Can you work these out from the model? Positions are in its coordinate system, mm. Face numbers are marked on the shaded views. A direction names the side the tool comes from. Round coordinates to 2 decimals unless told otherwise and drop trailing zeros. Write each loop counter-clockwise with the first axis right and the second up, starting at its lowest first coordinate (ties: lowest second). Pieces come first, ordered by that corner, then holes. Notation, with made-up numbers: M -31.5,-4.5 L 21.5,-4.5 A21 ccw 21.5,26.5 Z; hole C 56.25,59 d8. An arc over 180 degrees is marked long. Answer as a JSON object with one key per item and string values. Group by question number.
1) Suppose I cut it at C-C, the plane x = 2.25. Write out the boundary of the cut face in (y, z).
2) On a 3-axis mill with a long thin cutter (end or side, diameter ignored), from which of +Z, -Z, +X, -X, +Y, -Y can I reach the whole of each face in a straight line? I mean the marked faces 1 and 2. Say none if no direction works.
3) Suppose I cut it at D-D, the plane z = -1. Write out the boundary of the cut face in (x, y).
4) Please list where these lines run through material, in increasing order: L1, parallel to X at y = 0.75, z = -9.75; L2, parallel to Z at x = 2, y = 2.05; L3, parallel to Y at x = 8, z = -2.5. Write a range as [from, to].
5) Suppose I cut it at A-A, the plane z = -4.75. Write out the boundary of the cut face in (x, y).
6) Suppose I cut it at B-B, the plane x = 11.25. Write out the boundary of the cut face in (y, z), and give its area (3 significant figures).
7) I'm going to push flat-ended pins straight in: pin 1 Ø1.8 at (x, y) = (1, 2.5) entering from +Z; pin 2 Ø0.8 at (x, z) = (-0.5, -4.5) entering from -Y; pin 3 Ø5 at (x, z) = (10.5, -3.5) entering from +Y. Where does each tip first touch, or does it pass through?
from build123d import *

# Parameters (mm, degrees)
SKETCH1_R           = 0.5
SKETCH1_W           = 6.5
SKETCH1_H           = 9.1
BOSS_EXTRUDE1_DEPTH = 1
BOSS_EXTRUDE2_START = 1
SKETCH1_3_W         = 1
SKETCH1_3_H         = 9.1
SKETCH1_3_W_2       = 6.5
BOSS_EXTRUDE2_DEPTH = 3.2
FILLET1_R           = 1


with BuildPart() as part:
    # Sketch1 → Boss-Extrude1 (new body)
    # profile 1 of 2: a face of its own
    with BuildSketch(Plane(origin=(0, 0, 0), x_dir=(1, 0, 0), z_dir=(0, 1, 0))):
        Polygon((0, 1.45), (0, 0), (13.75, 0), (13.75, 12), (0, 12), (0, 10.55), (6.5, 10.55), (6.5, 1.45), align=None)
        with Locations(Location((11.25, 2.25, 0), (0, 0, 270))):
            Circle(SKETCH1_R, mode=Mode.SUBTRACT)
        with Locations(Location((11.25, 4.75, 0), (0, 0, 270))):
            Circle(SKETCH1_R, mode=Mode.SUBTRACT)
        with Locations(Location((11.25, 7.25, 0), (0, 0, 270))):
            Circle(SKETCH1_R, mode=Mode.SUBTRACT)
        with Locations(Location((11.25, 9.75, 0), (0, 0, 270))):
            Circle(SKETCH1_R, mode=Mode.SUBTRACT)
    # profile 2 of 2: a face of its own
    with BuildSketch(Plane(origin=(0, 0, 0), x_dir=(1, 0, 0), z_dir=(0, 1, 0))):
        with Locations((3.25, 6)):
            Rectangle(SKETCH1_W, SKETCH1_H)
    extrude(amount=BOSS_EXTRUDE1_DEPTH)

    # Sketch1<3> → Boss-Extrude2 (add)
    with BuildSketch(Plane(origin=(0, 0, 0), x_dir=(1, 0, 0), z_dir=(0, 1, 0)).offset(BOSS_EXTRUDE2_START)):
        with Locations((-0.5, 6)):
            Rectangle(SKETCH1_3_W, SKETCH1_3_H)
        with Locations((3.25, 6)):
            Rectangle(SKETCH1_3_W_2, SKETCH1_3_H)
    extrude(amount=BOSS_EXTRUDE2_DEPTH)

    # Fillet1
    fillet1_edges = [part.edges().sort_by_distance(p)[0] for p in [
        (2.75, 4.2, -10.55),
        (2.75, 4.2, -1.45),
    ]]
    fillet(fillet1_edges, radius=FILLET1_R)


solid = part.part
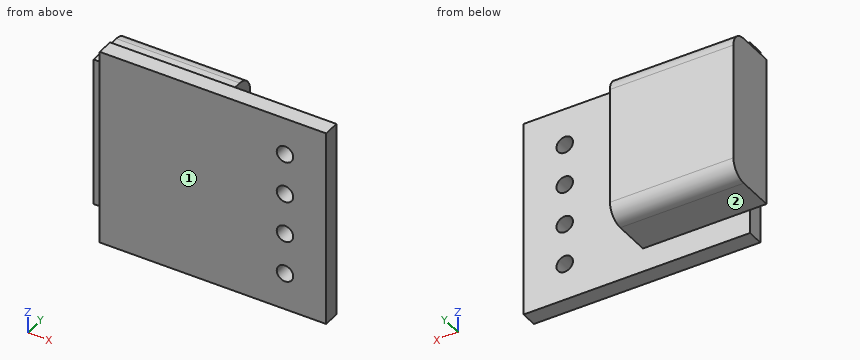
Results:
{
 "1": {"outline": "M 0,-12 L 1,-12 L 1,-10.55 L 3.2,-10.55 A1 ccw 4.2,-9.55 L 4.2,-2.45 A1 ccw 3.2,-1.45 L 1,-1.45 L 1,0 L 0,0 Z"},
 "2": {"face 1": "+Z, -Z, +X, -X, -Y", "face 2": "-Z, +X, -X, +Y"},
 "3": {"outline": "M 0,0 L 13.75,0 L 13.75,1 L 0,1 Z"},
 "4": {"L1": "[0, 10.75], [11.75, 13.75]", "L2": "[-10.55, -1.45]", "L3": "[0, 1]"},
 "5": {"outline": "M -1,1 L 0,1 L 0,0 L 10.75,0 L 10.75,1 L 6.5,1 L 6.5,4.2 L -1,4.2 Z; M 11.75,0 L 13.75,0 L 13.75,1 L 11.75,1 Z"},
 "6": {"outline": "M 0,-12 L 1,-12 L 1,-10.25 L 0,-10.25 Z; M 0,-9.25 L 1,-9.25 L 1,-7.75 L 0,-7.75 Z; M 0,-6.75 L 1,-6.75 L 1,-5.25 L 0,-5.25 Z; M 0,-4.25 L 1,-4.25 L 1,-2.75 L 0,-2.75 Z; M 0,-1.75 L 1,-1.75 L 1,0 L 0,0 Z", "area": "8.00 mm^2"},
 "7": {"pin 1": "z = -1.45", "pin 2": "y = 1", "pin 3": "y = 1"}
}
